Verification items for the finished model (mm, model axes). Face numbers are marked on the shaded views. A direction names the side the tool comes from. Coordinates: 2 decimals unless noted, no trailing zeros. Write each loop counter-clockwise with the first axis right and the second up, starting at its lowest first coordinate (ties: lowest second). Pieces come first, ordered by that corner, then holes. Notation, with made-up numbers: (22, -26.5) - (41, -26.5) arc R17 ccw to (41, -14.5) - close; hole circle Ø6 at (-17.75, 88.5). An arc over 180 degrees is marked (long way). Use one line per item in the form item = value. Start each with the question number.
(1) Sectioned sample at B-B (z = -7). Record the cut outline in (x, y), and give its area (3 significant figures).
(2) Tool access check on the marked faces 1, 2 and 3. Record the directions out of +Z, -Z, +X, -X, +Y, -Y that give a thin tool (end or side, any length) a straight path to the whole face; none if there is none.
(3) Sectioned sample at C-C (y = -3.25). Record the cut outline in (x, z), and give its area (3 significant figures).
(4) Gauge pin test, flat ends, axial feed: pin 1 Ø3 at (x, z) = (2.5, -6) entering from +Y; pin 2 Ø4.5 at (x, z) = (-2.5, -5.5) entering from -Y; pin 3 Ø1 at (x, z) = (-4, 2.5) entering from +Y (1 decimal); pin 4 Ø1.5 at (y, z) = (1.5, -5.5) entering from +X. Record the tip position at first contact, or that the pin passes through.
(5) Mould release check, pull along Y, two halves, no side actions. Record for the marked faces 4, 5, 6 and 7: released by +Y, released by -Y, zero draft, split by the parting line, or undercut.
(6) Sectioned sample at A-A (x = 0). Count the separate pieces of the cut face and the enclosed holes in it, and give its area (3 significant figures).
(7) Material ranges on line 1 (Z direction, x = 0, y = 4); line 2 (Y direction, x = 6.25, z = -4.75); line 3 (Z direction, x = 7.2, y = 0), recorded low to high. Write a range as [from, to].
(8) Sectioned sample at D-D (y = 1.25). Record the cut outline in (x, z), and give its area (3 significant figures).
from build123d import *

# Parameters (mm, degrees)
F0_R      = 8
F1_DEPTH  = 10
F3_DEPTH  = 10
F5_D      = 2
F5_DEPTH  = 8.001
F6_D      = 2
F7_R      = 2
F9_DEPTH  = 8
F10_R     = 1.9999
F11_R     = 1
F12_DEPTH = 8


# Not quite as in the source:
# - a fillet or chamfer is up to 0.001 mm smaller than in the source, because OpenCascade refuses the exact size
# - a feature names something its author has since deleted; it is built from what else it names


with BuildPart() as f1:
    # F0 (on Top) → F1 (new body, symmetric)
    with BuildSketch(Plane.XY):
        Circle(F0_R)
    extrude(amount=F1_DEPTH, both=True)

    # F2 (on face) → F3 (cut)
    with BuildSketch(Plane.XY.offset(10)):
        with BuildLine():
            ThreePointArc((5, 6.2449979984), (0, 8), (-5, 6.2449979984))
            Line((-5, 6.2449979984), (-5, -6.2449979984))
            ThreePointArc((-5, -6.2449979984), (0, -8), (5, -6.2449979984))
            Line((5, -6.2449979984), (5, 6.2449979984))
        make_face()
    extrude(amount=-F3_DEPTH, mode=Mode.SUBTRACT)

    # F5 (through all, one way)
    with BuildSketch(Plane.YZ):
        with Locations((0, 6)):
            Circle(F5_D / 2)
    extrude(amount=-F5_DEPTH, mode=Mode.SUBTRACT)

    # F6 (through all)
    with Locations(Plane(origin=(0, 0, 0), x_dir=(0, 1, 0), z_dir=(-1, 0, 0))):
        with Locations((0, -6)):
            Hole(F6_D / 2)

    # F7
    f7_edges = [f1.edges().sort_by_distance(p)[0] for p in [
        (5, 0, 10),
        (-5, 0, 10),
    ]]
    fillet(f7_edges, radius=F7_R)

    # F8 (on face) → F9 (cut)
    with BuildSketch(Plane(origin=(0, 0, -10), x_dir=(1, 0, 0), z_dir=(0, 0, -1))):
        with BuildLine():
            Line((7.7459666924, 2), (-7.7459666924, 2))
            ThreePointArc((-7.7459666924, 2), (-8, 0), (-7.7459666924, -2))
            Line((-7.7459666924, -2), (7.7459666924, -2))
            ThreePointArc((7.7459666924, -2), (7.9362375701, -1.0080343399), (8, 0))
            ThreePointArc((8, 0), (7.9362375701, 1.0080343399), (7.7459666924, 2))
        make_face()
    extrude(amount=-F9_DEPTH, mode=Mode.SUBTRACT)

    # F10 (radius 2 in the source; OpenCascade refuses exactly that, so slightly less here)
    f10_edges = [f1.edges().sort_by_distance(p)[0] for p in [
        (0, 2, -10),
        (0, -2, -10),
        (0, -2, -2),
        (0, 2, -2),
        (-5, 0, 0),
        (5, 0, 0),
    ]]
    fillet(f10_edges, radius=F10_R)

    # F11 (on Front) → F12 (cut, symmetric)
    with BuildSketch(Plane.XZ):
        with Locations((0, -7)):
            Circle(F11_R)
    extrude(amount=F12_DEPTH, both=True, mode=Mode.SUBTRACT)


solid = f1.part
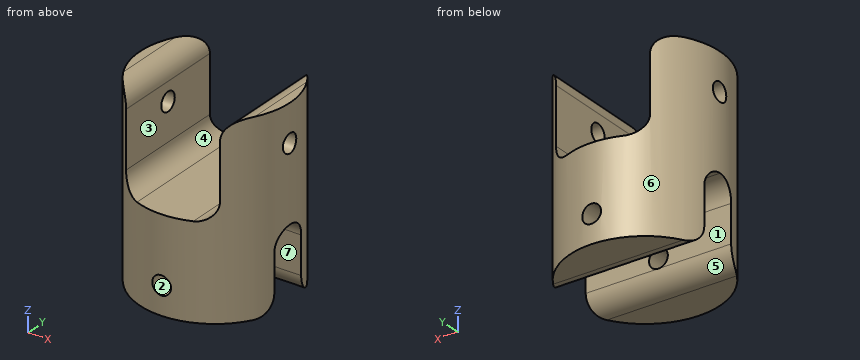
Answers below:
q1.outline = (-7.75, -2) arc R8 ccw to (-1, -7.94) - (-1, -2) - close; (-7.75, 2) - (-1, 2) - (-1, 7.94) arc R8 ccw to start; (1, -7.94) arc R8 ccw to (7.75, -2) - (1, -2) - close; (1, 2) - (7.75, 2) arc R8 ccw to (1, 7.94) - close
q1.area = 114 mm2
q2.face_1 = -Z, +X, -X
q2.face_2 = +Y, -Y
q2.face_3 = +Z, +Y, -Y
q3.outline = (-7.31, -9.85) - (7.31, -9.85) - (7.31, 10) - (7, 10) arc R2 ccw to (5, 8) - (5, 2) arc R2 cw to (3, 0) - (-3, 0) arc R2 cw to (-5, 2) - (-5, 8) arc R2 ccw to (-7, 10) - (-7.31, 10) - close; hole circle Ø2 at (0, -7)
q3.area = 187 mm2
q4.pin_1 = 7.94
q4.pin_2 = -8
q4.pin_3 = through
q4.pin_4 = 7.75
q5.face_4 = zero draft
q5.face_5 = undercut
q5.face_6 = split by the parting line
q5.face_7 = undercut
q6.separate_pieces = 3
q6.enclosed_holes = 0
q6.area = 104 mm2
q7.line_1 = [-10, -8], [-6, 0]
q7.line_2 = [-4.99, -2], [2, 4.99]
q7.line_3 = [-2, 5], [7, 10]
q8.outline = (-7.9, -2.44) - (7.9, -2.44) - (7.9, 10) - (7, 10) arc R2 ccw to (5, 8) - (5, 2) arc R2 cw to (3, 0) - (-3, 0) arc R2 cw to (-5, 2) - (-5, 8) arc R2 ccw to (-7, 10) - (-7.9, 10) - close
q8.area = 96.6 mm2
